Check sheet for the modelled part. Datum: model origin and axes. Units: mm. A direction names the side the tool comes from. Round coordinates to 2 decimals unless told otherwise and drop trailing zeros. Order: outer loops, then holes, each group sorted by start corner. A loop starts at its lowest first (then second) coordinate and runs counter-clockwise, first axis right, second up. Notation, with made-up numbers: (8, 80) -> (12, 80) arc R34 ccw to (12, 110) -> close; hole circle Ø11 at (47.5, 64). An arc over 180 degrees is marked (long way). Answer in a Markdown table with one row per item.
```python
from build123d import *

# Parameters (mm, degrees)
F0_R      = 38.1
F1_DEPTH  = 457.2
F3_R      = 25.4
F4_DEPTH  = 38.1
F1_FACE_R = 38.1
F4_FACE_R = 25.4


with BuildPart() as f1:
    # F0 (on Right) → F1 (new body, symmetric)
    with BuildSketch(Plane.YZ):
        Circle(F0_R)
    extrude(amount=F1_DEPTH, both=True)



with BuildPart() as f4:
    # F3 (on offset) → F4 (new body)
    with BuildSketch(Plane.YZ.offset(565.15)):
        Circle(F3_R)
    extrude(amount=F4_DEPTH)


with BuildPart() as f1_1:
    add(f1.part)

    add(f4.part)  # F5 merges F4
    # F1_face (on face) → F5 section 0
    with BuildSketch(Plane.YZ.offset(457.2)):
        Circle(F1_FACE_R)
    # F4_face (on face) → F5 section 1
    with BuildSketch(Plane(origin=(565.15, 0, 0), x_dir=(0, 1, 0), z_dir=(-1, 0, 0))):
        Circle(F4_FACE_R)
    loft()

    # F6: F1 across plane


with BuildPart() as f1_2:
    add(f1_1.part)
    add(f1_1.part.mirror(Plane.YZ))


solid = f1_2.part
```
(1) Tool access check on faces 1 (the cylindrical face through (583.933, -5.506, -24.796)), 2 (the cylindrical face through (-583.933, -5.506, -24.796)), 3 (the flat face through (603.25, 0, 0)). Record the directions out of +Z, -Z, +X, -X, +Y, -Y that give a thin tool (end or side, any length) a straight path to the whole face; none if there is none.
Solutions:
| item | result |
|---|---|
| face 1 | +X |
| face 2 | -X |
| face 3 | +Z, -Z, +X, +Y, -Y |
(2) Depth check by flat-ended pin: pin 1 Ø4 at (x, z) = (185.5, 24) entering from -Y; pin 2 Ø3 at (x, z) = (-316, 7.5) entering from +Y; pin 3 Ø2 at (x, z) = (299, 8) entering from +Y. Enter the tip coordinate at first touch or a pass-through.
Solutions:
| item | result |
|---|---|
| pin 1 | y = -31.11 |
| pin 2 | y = 37.62 |
| pin 3 | y = 37.45 |
(3) Section check A-A on y = 0. Record the boundary of the cut face in (x, z).
Solutions:
| item | result |
|---|---|
| outline | (-603.25, -25.4) -> (-565.15, -25.4) -> (-457.2, -38.1) -> (457.2, -38.1) -> (565.15, -25.4) -> (603.25, -25.4) -> (603.25, 25.4) -> (565.15, 25.4) -> (457.2, 38.1) -> (-457.2, 38.1) -> (-565.15, 25.4) -> (-603.25, 25.4) -> close |
(4) Scan lines: probe 1 along Z at (x, y) = (-86.5, -2); probe 2 along Z at (x, y) = (-518, -3); probe 3 along Y at (x, z) = (-423.5, 11.5). Record each from-to range of solid material in increasing order. Write a range as from..to.
Solutions:
| item | result |
|---|---|
| probe 1 | -38.05..38.05 |
| probe 2 | -30.8..30.8 |
| probe 3 | -36.32..36.32 |
(5) Section check B-B on x = -437. Record the boundary of the cut face in (y, z).
Solutions:
| item | result |
|---|---|
| outline | circle Ø76.2 at (0, 0) |
